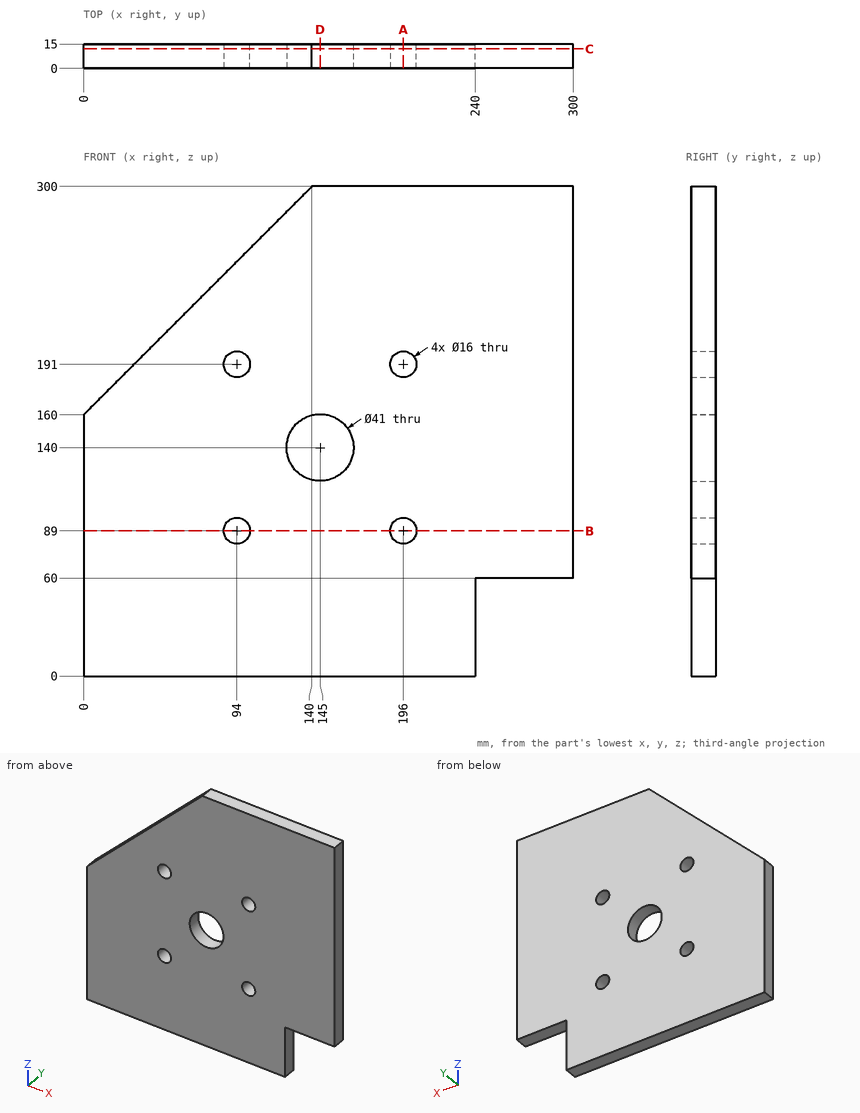
Here's the drawing with two shaded views (mm, measured from the low corner). I have some questions. Coordinates: 2 decimals unless noted, no trailing zeros. Write each loop counter-clockwise with the first axis right and the second up, starting at its lowest first coordinate (ties: lowest second). Pieces come first, ordered by that corner, then holes.
Item 1: I want a section at C-C on y = 12. Write out the boundary of the cut face in (x, z).
Item 2: I want a section at A-A on x = 196. Write out the boundary of the cut face in (y, z), and give its area (3 significant figures).
Item 3: I want a section at D-D on x = 145. Write out the boundary of the cut face in (y, z), and give its area (4 significant figures).
Item 4: If I drill on line 1 (Z direction, x = 196, y = 9); line 2 (X direction, y = 11.5, z = 90.5); line 3 (Z direction, x = 94, y = 5.5), over which ranges is the centre line in solid material (lowest first)?
Item 5: I want a section at B-B on z = 89. Write out the boundary of the cut face in (x, y).
Item 6: Will this pin go through, and if not, where does the flat tip stop? pin 1 (7.5 mm diameter, centred on y = 4, z = 39, fed in from +X).
Findings below:
1. outline: (0, 0) - (240, 0) - (240, 60) - (300, 60) - (300, 300) - (140, 300) - (0, 160) - close; hole circle Ø16 at (94, 89); hole circle Ø16 at (94, 191); hole circle Ø41 at (145, 140); hole circle Ø16 at (196, 89); hole circle Ø16 at (196, 191)
2. outline: (0, 0) - (15, 0) - (15, 81) - (0, 81) - close; (0, 97) - (15, 97) - (15, 183) - (0, 183) - close; (0, 199) - (15, 199) - (15, 300) - (0, 300) - close
2. area: 4,020 mm2
3. outline: (0, 0) - (15, 0) - (15, 119.5) - (0, 119.5) - close; (0, 160.5) - (15, 160.5) - (15, 300) - (0, 300) - close
3. area: 3,885 mm2
4. line 1: z = 0 to 81, 97 to 183, 199 to 300
4. line 2: x = 0 to 86.14, 101.86 to 188.14, 203.86 to 300
4. line 3: z = 0 to 81, 97 to 183, 199 to 254
5. outline: (0, 0) - (86, 0) - (86, 15) - (0, 15) - close; (102, 0) - (188, 0) - (188, 15) - (102, 15) - close; (204, 0) - (300, 0) - (300, 15) - (204, 15) - close
6. pin 1: stops at x = 240
